CAD build for the part. Positions are in the model's coordinates, mm. Face numbers are marked on the shaded views. Round coordinates to 2 decimals unless told otherwise and drop trailing zeros. Write each loop counter-clockwise with the first axis right and the second up, starting at its lowest first coordinate (ties: lowest second). Pieces come first, ordered by that corner, then holes. Notation, with made-up numbers: (29.25, 35.25) - (84.25, 35.25) arc R26 cw to (84.25, 49.25) - close; hole circle Ø5 at (2.25, 71). An arc over 180 degrees is marked (long way). Use one line per item in the form item = value. Start each with the question number.
Item 1: Drill centre lines: L1, parallel to Z at x = 13.5, y = 66.5; L2, parallel to Y at x = -113, z = 88; L3, parallel to X at y = 82, z = 167.5. Where is each one in solid material? Low to high.
Item 2: Pull direction Y, two halves, no side cores. Call the marked faces 1, 2, 3 and 4: +Y half, -Y half, draft (parallel to the pull), parting line (faces both ways), or undercut.
Item 3: Band-saw the part on B-B, the plane y = 59. List the corners of the cut face in (x, z).
Item 4: Band-saw the part on A-A, the plane x = -209. List the corners of the cut face in (y, z), and give its area (3 significant figures).
Item 5: Band-saw the part on C-C, the plane z = 117. List the corners of the cut face in (x, y), and give its area (3 significant figures).
Item 6: Pin check, flat tip, straight feed: pin 1 (6 mm diameter, centred on y = -65.5, z = 198.5, fed in from +X). Stop position of the tip, or through.
from build123d import *

# Parameters (mm, degrees)
F0_W      = 482.6
F0_H      = 228.6
F1_DEPTH  = 12.7
F1_FACE_W = 482.6
F1_FACE_H = 228.6
F2_DEPTH  = 114.3
F3_T      = -2.54


with BuildPart() as f1:
    # F0 (on Front) → F1 (new body, symmetric)
    with BuildSketch(Plane.XZ):
        with Locations((-108.143448, 114.3)):
            Rectangle(F0_W, F0_H)
    extrude(amount=F1_DEPTH, both=True)

    # F1_face (on face) + F0 (on Front) → F2 (join, symmetric)
    with BuildSketch(Plane(origin=(-108.143448, -12.7, 114.3), x_dir=(1, 0, 0), z_dir=(0, -1, 0))):
        Rectangle(F1_FACE_W, F1_FACE_H)
    with BuildSketch(Plane.XZ):
        with Locations((-108.143448, 114.3)):
            Rectangle(F0_W, F0_H)
    extrude(amount=F2_DEPTH, both=True)

    # F3
    f3_openings = [f1.faces().sort_by_distance(p)[0] for p in [
        (133.156552, -6.35, 114.3),
    ]]
    offset(amount=F3_T, openings=f3_openings)


solid = f1.part
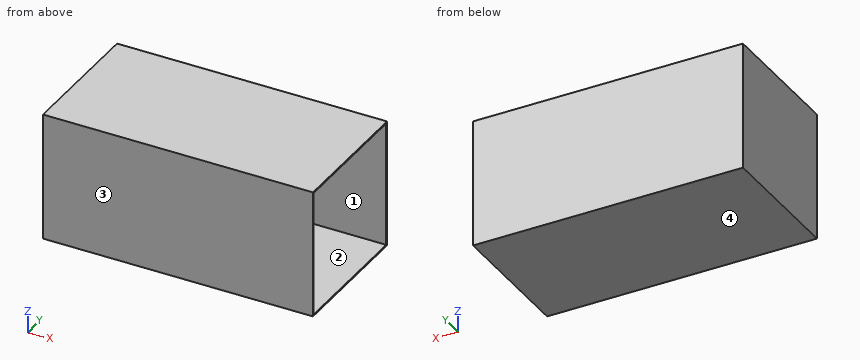
Determined:
q1.L1 = 0 to 2.54, 226.06 to 228.6
q1.L2 = -127 to -124.46, 111.76 to 114.3
q1.L3 = -349.44 to -346.9
q2.face_1 = undercut
q2.face_2 = undercut
q2.face_3 = -Y half
q2.face_4 = draft
q3.outline = (-349.44, 0) - (133.16, 0) - (133.16, 2.54) - (-346.9, 2.54) - (-346.9, 226.06) - (133.16, 226.06) - (133.16, 228.6) - (-349.44, 228.6) - close
q4.outline = (-127, 0) - (114.3, 0) - (114.3, 228.6) - (-127, 228.6) - close; hole (-124.46, 2.54) - (111.76, 2.54) - (111.76, 226.06) - (-124.46, 226.06) - close
q4.area = 2,360 mm²
q5.outline = (-349.44, -127) - (133.16, -127) - (133.16, -124.46) - (-346.9, -124.46) - (-346.9, 111.76) - (133.16, 111.76) - (133.16, 114.3) - (-349.44, 114.3) - close
q5.area = 3,050 mm²
q6.pin_1 = -346.9
